Source: three-view drawing plus pictorial views. Frame: mm from the lowest corner of the part. A direction names the side the tool comes from. Give positions to 0.01 mm unless a question says otherwise; leave off trailing zeros. Loops run counter-clockwise (first coordinate to the right, second up) from the corner with the lowest first, then second, coordinate; pieces in that order, holes last. Notation, with made-up numbers: M -32,-13 L -15,-13 A25 ccw -15,21 Z; hole C -27.75,-17 d2. An arc over 180 degrees is marked long. One line per item, written item: value. Start each with the question number.
(1) Section A-A on x = 6. Output: boundary loops of the cut face in (y, z).
(2) Section C-C on z = 20.5. Output: boundary loops of the cut face in (x, y), plus the area to 3 significant figures.
(3) Access query for the marked faces 1 and 2. Directions: +Z, -Z, +X, -X, +Y, -Y. A direction counts if a zero-diameter tool reaches every point of the face in a straight line with its end or side. Return the directions, or none.
(4) Section B-B on y = 6. Output: boundary loops of the cut face in (x, z).
(5) Pin query (flat end, axial travel): P1, Ø2, axis at y = 9.5, z = 20, coming from the +X side; P2, Ø5, axis at x = 5, z = 22, coming from the +Y side; P3, Ø5, axis at x = 9, z = 4.5, coming from the -Y side. Return the tip coordinate at first contact, or that it passes through.
(6) Ray query, line 1 along Z through (x, y) = (5, 1.25); line 2 along Z through (x, y) = (5, 5.5); line 3 along Y through (x, z) = (4.25, 23). Return the intervals inside material, ascending. Write a range as from..to.
(7) Section D-D on z = 13.25. Output: boundary loops of the cut face in (x, y).
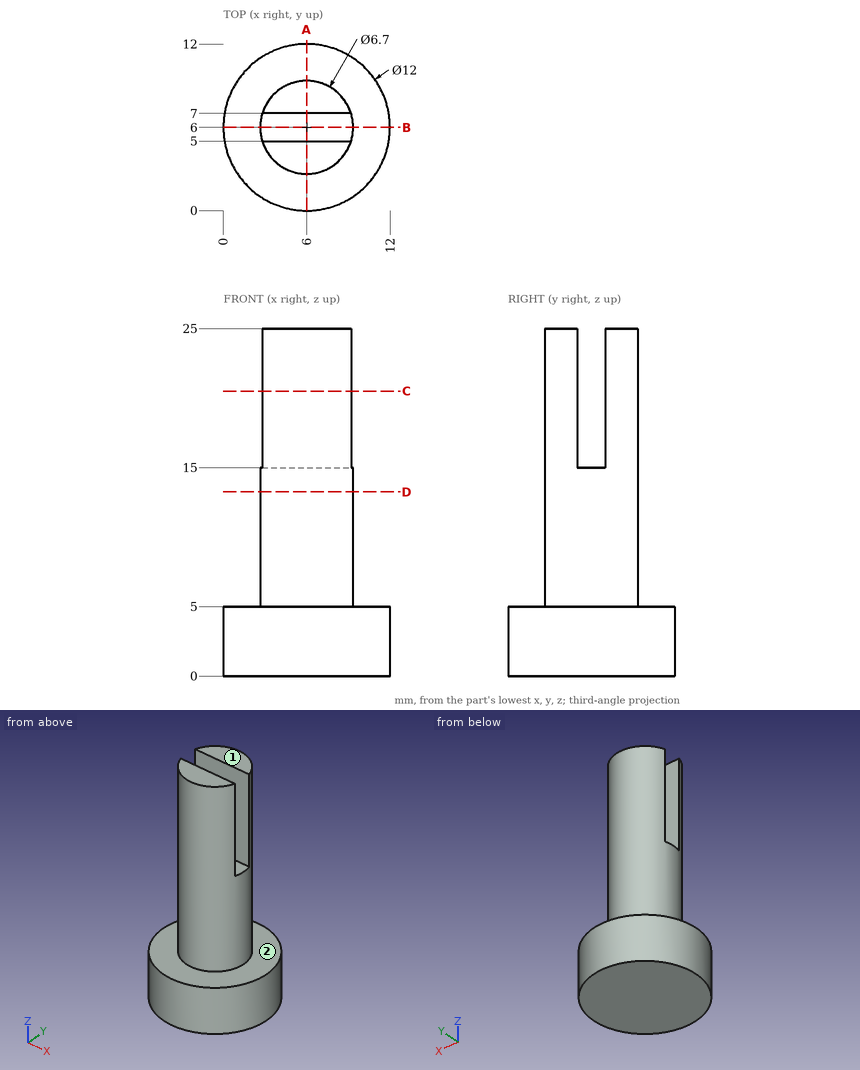
Output values:
1. outline: M 0,0 L 12,0 L 12,5 L 9.35,5 L 9.35,25 L 7,25 L 7,15 L 5,15 L 5,25 L 2.65,25 L 2.65,5 L 0,5 Z
2. outline: M 2.8,5 A3.35 ccw 9.2,5 Z; M 2.8,7 L 9.2,7 A3.35 ccw Z
2. area: 22.1 mm²
3. face 1: +Z, +X, -X, +Y, -Y
3. face 2: +Z
4. outline: M 0,0 L 12,0 L 12,5 L 9.35,5 L 9.35,15 L 2.65,15 L 2.65,5 L 0,5 Z
5. P1: stops at x = 8.23
5. P2: stops at y = 9.35
5. P3: stops at y = 0.02
6. line 1: z = 0..5
6. line 2: z = 0..15
6. line 3: y = 3.14..5, 7..8.86
7. outline: C 6,6 d6.7
